Design review of the part built by this model. Coordinates are the model's own, in mm. A direction names the side the tool comes from. Coordinates: 2 decimals unless noted, no trailing zeros. Write each loop counter-clockwise with the first axis right and the second up, starting at its lowest first coordinate (ties: lowest second). Pieces come first, ordered by that corner, then holes. Notation, with made-up numbers: M 66,2.25 L 70,2.25 A15 ccw 70,18.25 Z; hole C 73,-27 d4. An arc over 180 degrees is marked long. One line per question, with ' | ' between items.
from build123d import *

# Parameters (mm, degrees)
F0_W          = 101.6
F0_H          = 101.6
F1_DEPTH      = 101.6
F2_R          = 25.4
F3_DEPTH      = 101.6
F4_R          = 25.4
F5_DEPTH      = 101.6
F6_R          = 5.08
F8_R          = 25.4
F9_DEPTH      = 50.8
F9_DEPTH_BACK = 152.4


with BuildPart() as f1:
    # F0 (on Front) → F1 (new body)
    with BuildSketch(Plane.XZ):
        with Locations((50.8, 50.8)):
            Rectangle(F0_W, F0_H)
    extrude(amount=F1_DEPTH)

    # F2 (on face) → F3 (cut)
    with BuildSketch(Plane.XZ.offset(101.6)):
        with Locations((50.8, 50.8)):
            Circle(F2_R)
    extrude(amount=-F3_DEPTH, mode=Mode.SUBTRACT)

    # F4 (on face) → F5 (cut)
    with BuildSketch(Plane.YZ.offset(101.6)):
        with Locations((-50.8, 50.8)):
            Circle(F4_R)
    extrude(amount=-F5_DEPTH, mode=Mode.SUBTRACT)

    # F6
    f6_edges = [f1.edges().sort_by_distance(p)[0] for p in [
        (50.8, -101.6, 101.6),
        (101.6, -50.8, 101.6),
        (101.6, -101.6, 50.8),
        (50.8, -101.6, 0),
        (101.6, -50.8, 0),
        (101.6, 0, 50.8),
        (0, -50.8, 101.6),
        (50.8, 0, 101.6),
        (0, -50.8, 0),
        (50.8, 0, 0),
        (0, -101.6, 50.8),
        (0, 0, 50.8),
    ]]
    fillet(f6_edges, radius=F6_R)

    # F8 (on offset) → F9 (join, two sides)
    with BuildSketch(Plane.XZ.offset(101.6)) as f9_sk:
        Circle(F8_R)
    extrude(amount=F9_DEPTH)
    extrude(f9_sk.sketch, amount=-F9_DEPTH_BACK)


solid = f1.part
1. Take a section at C-C (y = -42). Write out the cut boundary in (x, z).
Answer sheet:
outline: M 0,25.4 A25.4 ccw long 25.4,0 L 96.52,0 A5.08 ccw 101.6,5.08 L 101.6,26.97 L 59.6,26.97 A25.4 cw 42,26.97 L 0,26.97 Z; M 0,74.63 L 42,74.63 A25.4 cw 59.6,74.63 L 101.6,74.63 L 101.6,96.52 A5.08 ccw 96.52,101.6 L 5.08,101.6 A5.08 ccw 0,96.52 Z
2. Draft analysis for pull direction X (two halves, no side actions). For faces 4 (the face through (0, -60, 76)), 5 (the face through (75.027, -20.111, 58.429)), 6 (the face through (0, -152.4, 0)), state which applies: pulls with the +X half, pulls with the -X half, needs draft (parallel to the pull), parting line crosses it, or undercut.
Answer sheet:
face 4: pulls with the -X half | face 5: undercut | face 6: needs draft
3. Take a section at B-B (x = 36). Write out the cut boundary in (y, z).
Answer sheet:
outline: M -101.6,5.08 A5.08 ccw -96.52,0 L -5.08,0 A5.08 ccw 0,5.08 L 0,30.16 L -36,30.16 A25.4 cw -65.6,30.16 L -101.6,30.16 Z; M -101.6,71.44 L -65.6,71.44 A25.4 cw -36,71.44 L 0,71.44 L 0,96.52 A5.08 ccw -5.08,101.6 L -96.52,101.6 A5.08 ccw -101.6,96.52 Z
4. Take a section at A-A (z = 50.8). Write out the cut boundary in (x, y), then the cut area to 3 significant figures.
Answer sheet:
outline: M 0,-96.52 A5.08 ccw 5.08,-101.6 L 25.4,-101.6 L 25.4,-76.2 L 0,-76.2 Z; M 0,-25.4 L 25.4,-25.4 L 25.4,0 L 5.08,0 A5.08 ccw 0,-5.08 Z; M 76.2,-101.6 L 96.52,-101.6 A5.08 ccw 101.6,-96.52 L 101.6,-76.2 L 76.2,-76.2 Z; M 76.2,-25.4 L 101.6,-25.4 L 101.6,-5.08 A5.08 ccw 96.52,0 L 76.2,0 Z | area: 2,560 mm^2
5. To check wall thickness, follow line 1 along Z through (x, y) = (27.5, -50.8); line 2 along Y through (x, z) = (79, 52); line 3 along Y through (x, z) = (53.5, 6.5). State the ranges of each line that lie inside material, in increasing order. Write a range as [from, to].
Answer sheet:
line 1: [0, 25.4], [76.2, 101.6] | line 2: [-101.6, -76.17], [-25.43, 0] | line 3: [-101.6, 0]
6. Tool access review of faces 1 (the face through (61.205, -1.528, 1.449)), 2 (the face through (60, -50, 0)), 3 (the face through (0, 50.8, 0)): name each direction out of +Z, -Z, +X, -X, +Y, -Y from which nothing blocks a thin tool from reaching the whole face with its end or side.
Answer sheet:
face 1: -Z, +X, +Y | face 2: -Z, +X, +Y, -Y | face 3: +Z, -Z, +X, -X, +Y
7. Take a section at D-D (z = 28). Write out the cut boundary in (x, y).
Answer sheet:
outline: M 0,-96.52 A5.08 ccw 5.08,-101.6 L 39.61,-101.6 L 39.61,-61.99 L 0,-61.99 Z; M 0,-39.61 L 39.61,-39.61 L 39.61,0 L 5.08,0 A5.08 ccw 0,-5.08 Z; M 61.99,-101.6 L 96.52,-101.6 A5.08 ccw 101.6,-96.52 L 101.6,-61.99 L 61.99,-61.99 Z; M 61.99,-39.61 L 101.6,-39.61 L 101.6,-5.08 A5.08 ccw 96.52,0 L 61.99,0 Z
8. Insertion check: pin 1 Ø2 at (x, y) = (11, -27.5) entering from -Z; pin 2 Ø3 at (x, z) = (60.5, 79) entering from -Y; pin 3 Ø10 at (x, y) = (36.5, -89) entering from -Z. Each pin has a flat end and moves straight along its axis. Give the tip position at first contact, or say it passes through.
Answer sheet:
pin 1: z = -23.35 | pin 2: y = -101.6 | pin 3: z = 0
